Work out the finished part from the listing and answer in its coordinate system (mm). Face numbers are marked on the shaded views. A direction names the side the tool comes from. Round coordinates to 2 decimals unless told otherwise and drop trailing zeros. Loops run counter-clockwise (first coordinate to the right, second up) from the corner with the lowest first, then second, coordinate; pieces in that order, holes last. Notation, with made-up numbers: (46, 67.5) - (59, 67.5) arc R27 cw to (59, 96.5) - close; hole circle Ø10 at (81.5, 16). An arc over 180 degrees is marked (long way). Answer as CSV lines item,"result". Start each with the question number.
```python
from build123d import *

# Parameters (mm, degrees)
SKETCH3_W               = 145
SKETCH3_H               = 20
BOSS_EXTRUDE3_DEPTH     = 45
BOSS_EXTRUDE6_DEPTH     = 60
CUT_EXTRUDE6_DEPTH      = 110.861912755
CUT_EXTRUDE6_DEPTH_BACK = 10
SKETCH10_W              = 60
SKETCH10_H              = 30
CUT_EXTRUDE7_DEPTH      = 90
CUT_EXTRUDE9_DEPTH      = 84
CUT_EXTRUDE9_DEPTH_BACK = 59
SKETCH11_R              = 12
SKETCH15_R              = 12
CUT_EXTRUDE10_DEPTH     = 40
SKETCH16_R              = 8
CUT_EXTRUDE11_DEPTH     = 40
FILLET1_R               = 20
FILLET2_R               = 20
FILLET3_R               = 20
FILLET4_R               = 20


with BuildPart() as part:
    # Sketch3 → Boss-Extrude3 (new, symmetric)
    with BuildSketch(Plane.XY):
        with Locations((12.618187605, -21.786578497)):
            Rectangle(SKETCH3_W, SKETCH3_H)
    extrude(amount=BOSS_EXTRUDE3_DEPTH, both=True)

    # Sketch4 → Boss-Extrude6 (add)
    with BuildSketch(Plane(origin=(0, -11.786578497, 0), x_dir=(1, 0, 0), z_dir=(0, 1, 0))):
        Polygon((5.118187605, 5), (-59.881812395, 5), (-59.881812395, -5), (5.118187605, -5), (5.118187605, 0), align=None)
        with BuildLine():
            Line((5.118187605, -30), (55.118187605, -30))
            ThreePointArc((55.118187605, -30), (85.118187605, 0), (55.118187605, 30))
            Line((55.118187605, 30), (5.118187605, 30))
            Line((5.118187605, 30), (5.118187605, 0))
            Line((5.118187605, 0), (5.118187605, -30))
        make_face()
    extrude(amount=BOSS_EXTRUDE6_DEPTH)

    # Sketch7 → Cut-Extrude6 (cut, two sides: drawn at the far end of the back side and taken through both)
    with BuildSketch(Plane.XY.offset(5).offset(-CUT_EXTRUDE6_DEPTH_BACK)):
        Polygon((-297.845774457, -231.445620401), (-59.881812395, -11.786578497), (5.118187605, 48.213421503), (243.082149668, 267.872463407), (-196.23593414, 743.800387532), (-737.163858265, 244.482303724), align=None)
    extrude(amount=CUT_EXTRUDE6_DEPTH + CUT_EXTRUDE6_DEPTH_BACK, mode=Mode.SUBTRACT)

    # Sketch10 → Cut-Extrude7 (cut)
    with BuildSketch(Plane.XY.offset(30)):
        with Locations((55.118187605, 18.213421503)):
            Rectangle(SKETCH10_W, SKETCH10_H)
    extrude(amount=-CUT_EXTRUDE7_DEPTH, mode=Mode.SUBTRACT)

    # Sketch11 → Cut-Extrude9 (cut, two sides: drawn at the far end of the back side and taken through both)
    with BuildSketch(Plane(origin=(0, 3.213421503, 0), x_dir=(1, 0, 0), z_dir=(0, 1, 0)).offset(-CUT_EXTRUDE9_DEPTH_BACK)):
        with Locations(Location((55.118187605, 0, 0), (0, 0, 90))):
            Circle(SKETCH11_R)
    extrude(amount=CUT_EXTRUDE9_DEPTH + CUT_EXTRUDE9_DEPTH_BACK, mode=Mode.SUBTRACT)

    # Sketch13 → Revolve1 (revolve)
    with BuildSketch(Plane.XY, mode=Mode.PRIVATE) as revolve1_sk:
        Polygon((55.118187605, 48.213421503), (55.118187605, 88.213421503), (35.118187605, 88.213421503), (25.118187605, 48.213421503), align=None)
    revolve(revolve1_sk.sketch.rotate(Axis((55.118187605, 48.213421503, 0), (0, 1, 0)), 90), axis=Axis((55.118187605, 48.213421503, 0), (0, 1, 0)))

    # Sketch15 → Cut-Extrude10 (cut)
    with BuildSketch(Plane(origin=(0, 88.213421503, 0), x_dir=(1, 0, 0), z_dir=(0, 1, 0))):
        with Locations(Location((55.118187605, 0, 0), (0, 0, 90))):
            Circle(SKETCH15_R)
    extrude(amount=-CUT_EXTRUDE10_DEPTH, mode=Mode.SUBTRACT)

    # Sketch16 → Cut-Extrude11 (cut)
    with BuildSketch(Plane(origin=(0, -11.786578497, 0), x_dir=(1, 0, 0), z_dir=(0, 1, 0))):
        with Locations(Location((-39.881812395, -25, 0), (0, 0, 270))):
            Circle(SKETCH16_R)
        with Locations(Location((-39.881812395, 25, 0), (0, 0, 270))):
            Circle(SKETCH16_R)
    extrude(amount=-CUT_EXTRUDE11_DEPTH, mode=Mode.SUBTRACT)

    # Fillet1
    fillet1_edges = [part.edges().sort_by_distance(p)[0] for p in [
        (-59.881812395, -21.786578497, 45),
    ]]
    fillet(fillet1_edges, radius=FILLET1_R)

    # Fillet2
    fillet2_edges = [part.edges().sort_by_distance(p)[0] for p in [
        (-59.881812395, -21.786578497, -45),
    ]]
    fillet(fillet2_edges, radius=FILLET2_R)

    # Fillet3
    fillet3_edges = [part.edges().sort_by_distance(p)[0] for p in [
        (85.118187605, -21.786578497, -45),
    ]]
    fillet(fillet3_edges, radius=FILLET3_R)

    # Fillet4
    fillet4_edges = [part.edges().sort_by_distance(p)[0] for p in [
        (85.118187605, -21.786578497, 45),
    ]]
    fillet(fillet4_edges, radius=FILLET4_R)


solid = part.part
```
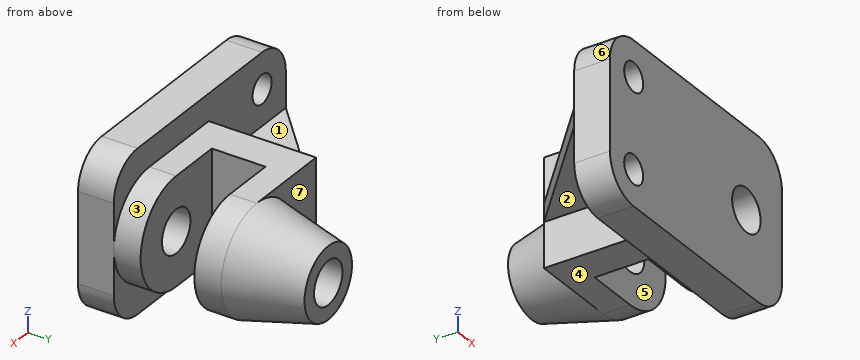
Item 1: Flat-ended cylindrical pins translate along their axes: pin 1 Ø6 at (x, z) = (15.5, -20) entering from +Y; pin 2 Ø7.5 at (y, z) = (24.5, 12.5) entering from -X; pin 3 Ø1.5 at (x, y) = (25, 3.5) entering from -Z. Find the tip coordinate at first contact, or state that the pin passes through.
Item 2: Determine the mould class of the marked faces 5, 6 and 7 for opening direction Y: pulls with the +Y half, pulls with the -Y half, needs draft (parallel to the pull), parting line crosses it, or undercut.
Item 3: Which of the six approach directions +Z, -Z, +X, -X, +Y, -Y give full straight-line access (tool end or side, diameter ignored) to the marked faces 1, 2, 3 and 4?
Item 4: Section C-C, the plane y = 35.5 is taken. Give the vertices of the cut face in (x, z).
Item 5: Find the intervals of material crossed by L1, parallel to Y at x = 73, z = -7; L2, parallel to Y at x = 27.5, z = 27.5; L3, parallel to Z at x = -32.5, y = -18, in increasing order.
Item 6: Section A-A, the plane x = 15 is taken. Give the vertices of the cut face in (y, z).
Item 7: Section B-B, the plane y = 7 is taken. Give the vertices of the cut face in (x, z).
Item 8: Section D-D, the plane z = -9.5 is taken. Count the separate pieces of the cut face and the enclosed holes in it, and give its area (3 significant figures).
Answer:
1,pin 1,"stops at y = 48.21"
1,pin 2,"stops at x = 5.12"
1,pin 3,"stops at z = -30"
2,face 5,"undercut"
2,face 6,"needs draft"
2,face 7,"pulls with the +Y half"
3,face 1,"+Z, -X, +Y"
3,face 2,"-Z, -X, +Y"
3,face 3,"+X, +Y"
3,face 4,"-Z, +X, -X, +Y"
4,outline,"(-8.65, -5) - (5.12, -5) - (5.12, -30) - (55.12, -30) arc R30 ccw to (55.12, 30) - (5.12, 30) - (5.12, 5) - (-8.65, 5) - close; hole circle Ø24 at (55.12, 0)"
5,L1,"y = -31.79 to 3.21, 33.21 to 88.21"
5,L2,"y = -31.79 to 3.21, 33.21 to 48.21"
5,L3,"z = -45 to -28.08, -21.92 to 21.92, 28.08 to 45"
6,outline,"(-31.79, -45) - (-11.79, -45) - (-11.79, -30) - (48.21, -30) - (48.21, 30) - (-11.79, 30) - (-11.79, 45) - (-31.79, 45) - close"
7,outline,"(-39.53, -5) - (5.12, -5) - (5.12, -30) - (25.12, -30) - (25.12, 30) - (5.12, 30) - (5.12, 5) - (-39.53, 5) - close"
8,separate pieces,"3"
8,enclosed holes,"0"
8,area,"6,380 mm²"
